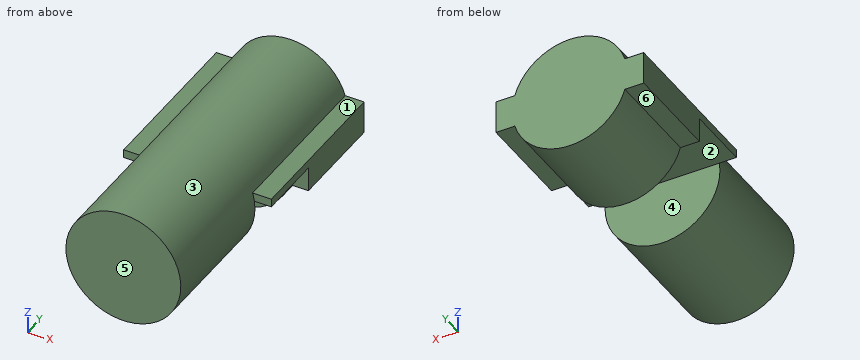
from build123d import *

# Parameters (mm, degrees)
SKETCH1_R           = 3.5
BOSS_EXTRUDE1_DEPTH = 18
SKETCH2_W           = 9
SKETCH2_H           = 2
BOSS_EXTRUDE3_DEPTH = 10
CUT_EXTRUDE3_START  = -8
SKETCH3_W           = 10
SKETCH3_H           = 4
CUT_EXTRUDE3_DEPTH  = 4


with BuildPart() as part:
    # Sketch1 → Boss-Extrude1 (new body)
    with BuildSketch(Plane(origin=(0, 0, 0), x_dir=(1, 0, 0), z_dir=(0, 1, 0))):
        with Locations(Location((0, 0, 0), (0, 0, 270))):
            Circle(SKETCH1_R)
    extrude(amount=BOSS_EXTRUDE1_DEPTH)

    # Sketch2 → Boss-Extrude3 (add)
    with BuildSketch(Plane(origin=(0, 18, 0), x_dir=(1, 0, 0), z_dir=(0, 1, 0))):
        Rectangle(SKETCH2_W, SKETCH2_H)
    extrude(amount=-BOSS_EXTRUDE3_DEPTH)

    # Sketch3 → Cut-Extrude3 (cut)
    with BuildSketch(Plane.XZ.offset(CUT_EXTRUDE3_START)):
        with Locations((0, -1.5)):
            Rectangle(SKETCH3_W, SKETCH3_H)
    extrude(amount=-CUT_EXTRUDE3_DEPTH, mode=Mode.SUBTRACT)


solid = part.part
Read the model definition and answer for the solid it produces. Units are mm, in the model's axes. Face numbers are marked on the shaded views. A direction names the side the tool comes from. Coordinates: 2 decimals unless noted, no trailing zeros. Loops run counter-clockwise (first coordinate to the right, second up) from the corner with the lowest first, then second, coordinate; pieces in that order, holes last. Notation, with made-up numbers: (22.25, 17) - (71.25, 17) arc R18 cw to (71.25, 51) - close; hole circle Ø3 at (-2.5, 79.25). An arc over 180 degrees is marked (long way). Answer in a Markdown table with one row per item.
Q1. For the marked faces 1, 2 and 3, determine the directions among +Z, -Z, +X, -X, +Y, -Y from which every point of the face is accessible in a straight line to the end or side of a thin tool.
Here are the results:
| item | result |
|---|---|
| face 1 | +Z, +X, +Y, -Y |
| face 2 | -Z, +X, -X |
| face 3 | -Y |
Q2. Find section D-D on z = -1.25. Write down the section's boundary in (x, y).
Here are the results:
| item | result |
|---|---|
| outline | (-3.27, 0) - (3.27, 0) - (3.27, 8) - (-3.27, 8) - close; (-3.27, 12) - (3.27, 12) - (3.27, 18) - (-3.27, 18) - close |
Q3. Find section C-C on x = 0. Write down the section's boundary in (y, z), plus the area to 3 significant figures.
Here are the results:
| item | result |
|---|---|
| outline | (0, -3.5) - (8, -3.5) - (8, 0.5) - (12, 0.5) - (12, -3.5) - (18, -3.5) - (18, 3.5) - (0, 3.5) - close |
| area | 110 mm^2 |
Q4. Given P1, Ø3, axis at y = 3.5, z = -2, coming from the +X side; P2, Ø1.5, axis at x = -0.5, y = 5, coming from the -Z side; P3, Ø0.6, axis at x = -4, y = 15, coming from the -Z side; P4, Ø2, axis at x = -3, y = 6.5, coming from the +Z side, each flat-ended and moving along its own axis, determine where each tip first touches the part or whether it passes through.
Here are the results:
| item | result |
|---|---|
| P1 | stops at x = 3.46 |
| P2 | stops at z = -3.5 |
| P3 | stops at z = -1 |
| P4 | stops at z = 2.87 |
Q5. The mould has two halves that part along Y. Classify the marked faces 4, 5 and 6: pulls with the +Y half, pulls with the -Y half, needs draft (parallel to the pull), parting line crosses it, or undercut.
Here are the results:
| item | result |
|---|---|
| face 4 | undercut |
| face 5 | pulls with the -Y half |
| face 6 | needs draft |
Q6. Straight lines are drawn through the part: line 1 along Y through (x, z) = (0.5, -1); line 2 along Y through (x, z) = (3.5, -0.5); line 3 along Z through (x, y) = (1, 1.75). For each, find the intervals that lie inside material, in ascending order. Write a range as [from, to].
Here are the results:
| item | result |
|---|---|
| line 1 | y = [0, 8], [12, 18] |
| line 2 | y = [12, 18] |
| line 3 | z = [-3.35, 3.35] |
Q7. Find section B-B on y = 15. Write down the section's boundary in (x, z).
Here are the results:
| item | result |
|---|---|
| outline | (-4.5, -1) - (-3.35, -1) arc R3.5 ccw to (3.35, -1) - (4.5, -1) - (4.5, 1) - (3.35, 1) arc R3.5 ccw to (-3.35, 1) - (-4.5, 1) - close |
Q8. Find section A-A on z = 0. Write down the section's boundary in (x, y), plus the area to 3 significant figures.
Here are the results:
| item | result |
|---|---|
| outline | (-4.5, 12) - (4.5, 12) - (4.5, 18) - (-4.5, 18) - close; (-3.5, 0) - (3.5, 0) - (3.5, 8) - (-3.5, 8) - close |
| area | 110 mm^2 |
